Design review of the part built by this model. Coordinates are the model's own, in mm. A direction names the side the tool comes from. Give positions to 0.01 mm unless a question says otherwise; leave off trailing zeros. Loops run counter-clockwise (first coordinate to the right, second up) from the corner with the lowest first, then second, coordinate; pieces in that order, holes last. Notation, with made-up numbers: (-10, -4) -> (-3, -4) arc R10 ccw to (-3, 2) -> close; hole circle Ø5 at (46.5, 19.25). An arc over 180 degrees is marked (long way). Answer in a Markdown table with one row per item. Add a question column.
(1) Consider section A-A on y = 7.25. Write out the cut boundary in (x, z).
(2) For faces 1 (the cylindrical face through (0, 4, -3)), 2 (the flat face through (0, 0, 0)), list the 3-axis set-ups (+Z, -Z, +X, -X, +Y, -Y) from which the entire face can be reached by the end or side of a thin tool; tool diameter is ignored.
(3) For pin 1 (10 mm diameter, centred on x = 4.5, z = 5.5, fed in from +Y); pin 2 (2 mm diameter, centred on x = 1, z = -1, fed in from -Y); pin 3 (0.7 mm diameter, centred on y = 4, z = 0, fed in from +X), all flat-tipped, find the tip position at first contact; note any pin that passes through.
(4) For line 1 (Z direction, x = 0, y = 3.5); line 2 (X direction, y = 8.15, z = 0); line 3 (X direction, y = 5.5, z = -2) (3 decimals), list the stretches that pass through material, from the lowest coordinate up.
(5) Draft analysis for pull direction X (two halves, no side actions). For faces 3 (the flat face through (10, 8.6, 11)), 4 (the flat face through (0, 4, 2.1)), 5 (the cylindrical face through (-3.512, 7.586, 15.815)), state which applies: +X half, -X half, draft (parallel to the pull), parting line (faces both ways), or undercut.
from build123d import *

# Parameters (mm, degrees)
SKETCH1_R           = 14.1
BUTTON_TOP_DEPTH    = 1.8
SKETCH2_R           = 14.1
SKETCH2_R_2         = 12.3
BUTTON_WALLS_DEPTH  = 4.8
SKETCH5_R           = 5
OFFSET_2_DEPTH      = 0.2
STEM_START          = 0.2
STEM_HOUSING_DEPTH  = 4.6
CHAMFER1_SIZE       = 1.5
FILLET2_R           = 1
SKETCH8_R           = 16.2
SKETCH8_R_2         = 14.3
BOSS_EXTRUDE1_DEPTH = 2


with BuildPart() as part:
    # Sketch1 → button top (new body)
    with BuildSketch(Plane(origin=(0, 0, 0), x_dir=(1, 0, 0), z_dir=(0, 1, 0))):
        Circle(SKETCH1_R)
    extrude(amount=BUTTON_TOP_DEPTH)

    # Sketch2 → button walls (add)
    with BuildSketch(Plane(origin=(0, 1.8, 0), x_dir=(1, 0, 0), z_dir=(0, 1, 0))):
        Circle(SKETCH2_R)
        Circle(SKETCH2_R_2, mode=Mode.SUBTRACT)
    extrude(amount=BUTTON_WALLS_DEPTH)

    # Sketch5 → offset 2 (add)
    with BuildSketch(Plane(origin=(0, 1.8, 0), x_dir=(1, 0, 0), z_dir=(0, 1, 0))):
        Circle(SKETCH5_R)
    extrude(amount=OFFSET_2_DEPTH)

    # Sketch3 → stem housing (add)
    with BuildSketch(Plane(origin=(0, 1.8, 0), x_dir=(1, 0, 0), z_dir=(0, 1, 0)).offset(STEM_START)):
        with BuildLine():
            Line((-3.6, 2.6), (-3.6, -2.6))
            Line((-3.6, -2.6), (-1.496662955, -2.6))
            ThreePointArc((-1.496662955, -2.6), (-3, 0), (-1.496662955, 2.6))
            Line((-1.496662955, 2.6), (-3.6, 2.6))
        make_face()
        with BuildLine():
            ThreePointArc((-1.496662955, 2.6), (-3, 0), (-1.496662955, -2.6))
            Line((-1.496662955, -2.6), (1.496662955, -2.6))
            ThreePointArc((1.496662955, -2.6), (2.597112711, -1.501667596), (3, 0))
            ThreePointArc((3, 0), (2.597112711, 1.501667596), (1.496662955, 2.6))
            Line((1.496662955, 2.6), (-1.496662955, 2.6))
        make_face()
        with BuildLine():
            ThreePointArc((-0.975, 0.675), (-0.762867966, 0.762867966), (-0.675, 0.975))
            Line((-0.675, 0.975), (-0.675, 2.1))
            Line((-0.675, 2.1), (0.675, 2.1))
            Line((0.675, 2.1), (0.675, 0.975))
            ThreePointArc((0.675, 0.975), (0.762867966, 0.762867966), (0.975, 0.675))
            Line((0.975, 0.675), (2.1, 0.675))
            Line((2.1, 0.675), (2.1, -0.675))
            Line((2.1, -0.675), (0.975, -0.675))
            ThreePointArc((0.975, -0.675), (0.762867966, -0.762867966), (0.675, -0.975))
            Line((0.675, -0.975), (0.675, -2.1))
            Line((0.675, -2.1), (-0.675, -2.1))
            Line((-0.675, -2.1), (-0.675, -0.975))
            ThreePointArc((-0.675, -0.975), (-0.762867966, -0.762867966), (-0.975, -0.675))
            Line((-0.975, -0.675), (-2.1, -0.675))
            Line((-2.1, -0.675), (-2.1, 0.675))
            Line((-2.1, 0.675), (-0.975, 0.675))
        make_face(mode=Mode.SUBTRACT)
        with BuildLine():
            ThreePointArc((3, 0), (2.597112711, -1.501667596), (1.496662955, -2.6))
            Line((1.496662955, -2.6), (3.6, -2.6))
            Line((3.6, -2.6), (3.6, 2.6))
            Line((3.6, 2.6), (1.496662955, 2.6))
            ThreePointArc((1.496662955, 2.6), (2.597112711, 1.501667596), (3, 0))
        make_face()
        with BuildLine():
            ThreePointArc((1.496662955, 2.6), (0, 3), (-1.496662955, 2.6))
            Line((-1.496662955, 2.6), (1.496662955, 2.6))
        make_face()
        with BuildLine():
            Line((1.496662955, -2.6), (-1.496662955, -2.6))
            ThreePointArc((-1.496662955, -2.6), (0, -3), (1.496662955, -2.6))
        make_face()
    extrude(amount=STEM_HOUSING_DEPTH)

    # Chamfer1
    chamfer1_edges = [part.edges().sort_by_distance(p)[0] for p in [
        (-12.3, 6.6, 0),
    ]]
    chamfer(chamfer1_edges, length=CHAMFER1_SIZE)

    # Fillet2
    fillet2_edges = [part.edges().sort_by_distance(p)[0] for p in [
        (-3.6, 4.3, -2.6),
        (-3.6, 4.3, 2.6),
        (3.6, 4.3, 2.6),
        (3.6, 4.3, -2.6),
    ]]
    fillet(fillet2_edges, radius=FILLET2_R)

    # Sketch6 → Cut-Revolve1 (revolve, cut)
    with BuildSketch(Plane.XY):
        with BuildLine():
            Line((-13.361522369, 0), (-13.561522369, 0.2))
            ThreePointArc((-13.561522369, 0.2), (-13.960054223, 0.79644507), (-14.1, 1.5))
            Line((-14.1, 1.5), (-14.1, 0))
            Line((-14.1, 0), (-13.361522369, 0))
        make_face()
    revolve(axis=Axis((0, 0, 0), (0, 1, 0)), mode=Mode.SUBTRACT)

    # Sketch7 → Revolve1 (revolve)
    with BuildSketch(Plane.XY):
        Polygon((14.1, 6.6), (15.7, 6.6), (14.1, 5), align=None)
    revolve(axis=Axis((0, 0, 0), (0, 1, 0)))

    # Sketch8 → Boss-Extrude1 (add)
    with BuildSketch(Plane(origin=(0, 6.6, 0), x_dir=(1, 0, 0), z_dir=(0, 1, 0))):
        Circle(SKETCH8_R)
        Circle(SKETCH8_R_2, mode=Mode.SUBTRACT)
    extrude(amount=BOSS_EXTRUDE1_DEPTH)


solid = part.part
Values follow:
| question | item | result |
|---|---|---|
| 1 | outline | circle Ø32.4 at (0, 0); hole circle Ø28.6 at (0, 0) |
| 2 | face 1 | +Y |
| 2 | face 2 | +Z, -Z, +X, -X, -Y |
| 3 | pin 1 | y = 6.6 |
| 3 | pin 2 | y = 0 |
| 3 | pin 3 | x = 14.1 |
| 4 | line 1 | -14.1 to -12.3, -3 to -2.1, 2.1 to 3, 12.3 to 14.1 |
| 4 | line 2 | -16.2 to -14.3, 14.3 to 16.2 |
| 4 | line 3 | -14.462 to -12.542, -3.517 to -0.675, 0.675 to 3.517, 12.542 to 14.462 |
| 5 | face 3 | draft |
| 5 | face 4 | undercut |
| 5 | face 5 | parting line |
